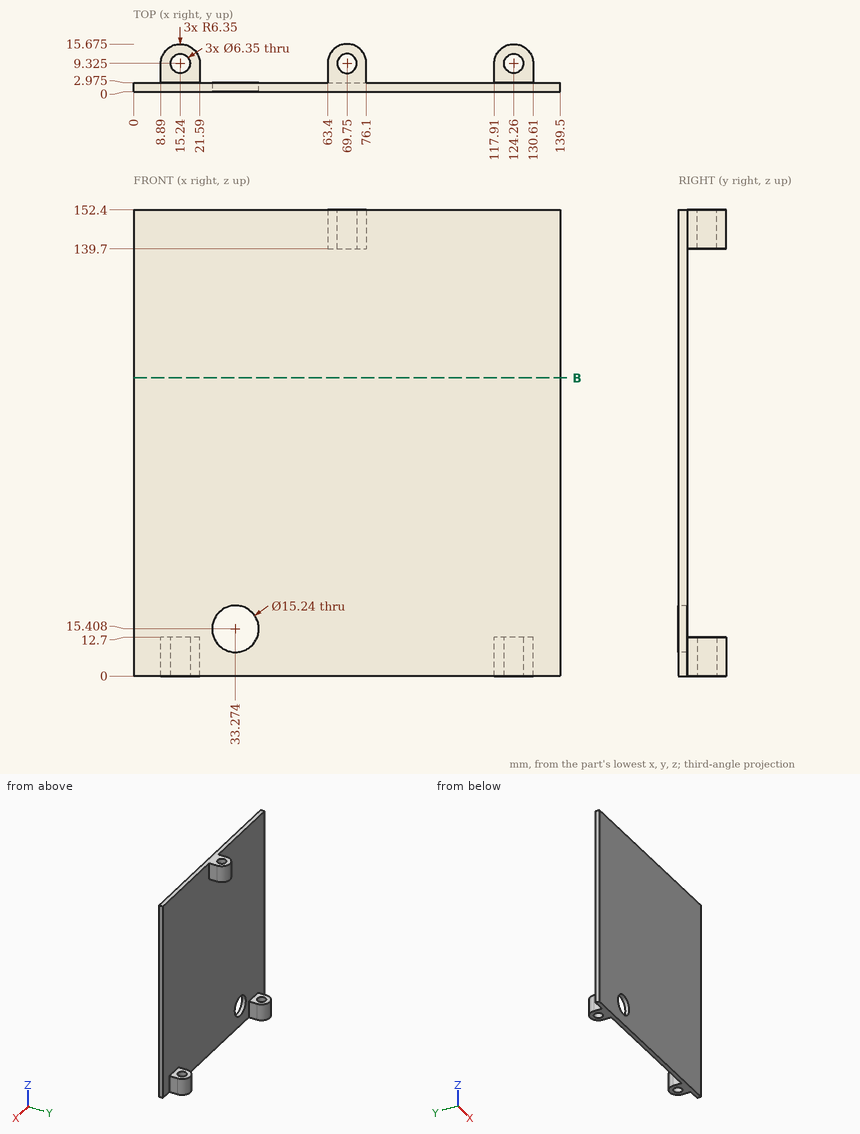
Answer from the drawing. Dimensions are ordinates in mm from the lowest x, y and z of the part. Round coordinates to 2 decimals unless told otherwise and drop trailing zeros. Order: outer loops, then holes, each group sorted by start corner. A loop starts at its lowest first (then second) coordinate and runs counter-clockwise, first axis right, second up.
1) Straight lines are drawn through the part: L1, parallel to Y at x = 15, z = 8; L2, parallel to Y at x = 90.5, z = 111 (1 decimal); L3, parallel to Z at x = 70.5, y = 4. For each, find the intervals that lie inside material, in ascending order.
2) The part is cut by section B-B on z = 97.5. Write down the section's boundary in (x, y) (1 decimal), plus the area to 3 significant figures.
3) Flat-ended cylindrical pins translate along their axes: pin 1 (6 mm diameter, centred on x = 47.5, z = 126.5, fed in from +Y) (3 decimals); pin 2 (7.5 mm diameter, centred on x = 15.24, y = 9.325, fed in from +Z); pin 3 (7 mm diameter, centred on y = 7.5, z = 148, fed in from +X). Find the tip coordinate at first contact, or state that the pin passes through.
Resolved:
1. L1: y = 0 to 6.16, 12.49 to 15.67
1. L2: y = 0 to 3
1. L3: z = 139.7 to 152.4
2. outline: (0, 0) - (139.5, 0) - (139.5, 3) - (0, 3) - close
2. area: 415 mm2
3. pin 1: stops at y = 2.975
3. pin 2: stops at z = 12.7
3. pin 3: stops at x = 76.1
